```python
from build123d import *

# Parameters (mm, degrees)
BOSS_EXTRUDE1_DEPTH = 13.7
SKETCH3_W           = 0.178571672
SKETCH3_H           = 6.380917094
CUT_EXTRUDE1_DEPTH  = 0.2
SKETCH4_R           = 0.85
BOSS_EXTRUDE3_DEPTH = 1.8
SKETCH5_W           = 0.138137893
SKETCH5_H           = 1.329179466
BOSS_EXTRUDE4_DEPTH = 2.8
SKETCH6_R           = 0.20198457
CUT_EXTRUDE2_DEPTH  = 9.6


with BuildPart() as part:
    # Sketch1 → Boss-Extrude1 (new body)
    with BuildSketch(Plane.XY):
        with BuildLine():
            Line((-3.31662479, -5), (3.31662479, -5))
            ThreePointArc((3.31662479, -5), (6, 0), (3.31662479, 5))
            Line((3.31662479, 5), (-3.31662479, 5))
            ThreePointArc((-3.31662479, 5), (-6, 0), (-3.31662479, -5))
        make_face()
    extrude(amount=BOSS_EXTRUDE1_DEPTH)

    # Sketch3 → Cut-Extrude1 (cut)
    with BuildSketch(Plane(origin=(0, 5, 0), x_dir=(1, 0, 0), z_dir=(0, 1, 0))):
        with Locations((-2.495957535, -5.684471075)):
            Rectangle(SKETCH3_W, SKETCH3_H)
        with Locations((2.495957535, -5.684471075)):
            Rectangle(SKETCH3_W, SKETCH3_H)
    extrude(amount=-CUT_EXTRUDE1_DEPTH, mode=Mode.SUBTRACT)

    # Sketch4 → Boss-Extrude3 (add)
    with BuildSketch(Plane(origin=(0, 0, 0), x_dir=(-1, 0, 0), z_dir=(0, 0, -1))):
        with Locations(Location((0, 0, 0), (0, 0, 180))):
            Circle(SKETCH4_R)
    extrude(amount=BOSS_EXTRUDE3_DEPTH)

    # Sketch5 → Boss-Extrude4 (add)
    with BuildSketch(Plane(origin=(0, 0, 0), x_dir=(-1, 0, 0), z_dir=(0, 0, -1))):
        with Locations((-4.217525365, 0)):
            Rectangle(SKETCH5_W, SKETCH5_H)
        with Locations((4.217525365, 0)):
            Rectangle(SKETCH5_W, SKETCH5_H)
    extrude(amount=BOSS_EXTRUDE4_DEPTH)

    # Sketch6 → Cut-Extrude2 (cut)
    with BuildSketch(Plane.ZY.offset(4.286594311)):
        with Locations((-2.171650698, 0)):
            Circle(SKETCH6_R)
    extrude(amount=-CUT_EXTRUDE2_DEPTH, mode=Mode.SUBTRACT)


solid = part.part
```
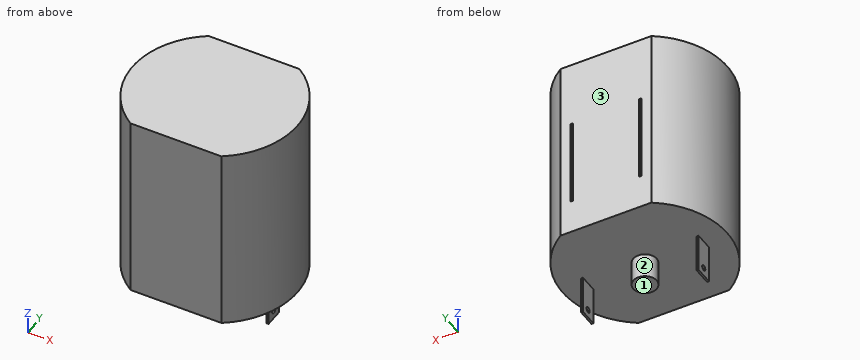
The listing builds one solid part. Answer for the finished solid, in the listing's coordinates (mm). Face numbers are marked on the shaded views. A direction names the side the tool comes from. Coordinates: 2 decimals unless noted, no trailing zeros. Loops run counter-clockwise (first coordinate to the right, second up) from the corner with the lowest first, then second, coordinate; pieces in that order, holes last. Notation, with made-up numbers: (-29, -17) - (-9, -17) arc R28 cw to (-9, 22) - close; hole circle Ø5 at (-35, 17). An arc over 180 degrees is marked (long way). Use a Markdown table: item, result. Add a question column.
1) Find the intervals of material crossed by line 1 (Z direction, x = 0, y = -3); line 2 (Y direction, x = 5, z = 3.5); line 3 (X direction, y = -3.5, z = 6), in increasing order.
2) The part is cut by section A-A, the plane y = 0. Give the vertices of the cut face in (x, z), and give its area (3 significant figures).
3) The part is cut by section B-B, the plane x = 0. Give the vertices of the cut face in (y, z).
4) The part is cut by section C-C, the plane z = 5.25. Give the vertices of the cut face in (x, y), and give its area (3 significant figures).
5) The part is cut by section D-D, the plane y = -1.5. Give the vertices of the cut face in (x, z).
6) For the marked faces 1, 2 and 3, determine the directions among +Z, -Z, +X, -X, +Y, -Y from which every point of the face is accessible in a straight line to the end or side of a thin tool.
7) Given pin 1 (1 mm diameter, centred on x = -3, y = -1.5, fed in from -Z); pin 2 (1.1 mm diameter, centred on y = 0, z = -1, fed in from +X); pin 3 (5 mm diameter, centred on x = -1, y = -0.5, fed in from -Z), each flat-ended and moving along its own axis, determine where each tip first touches the part or whether it passes through.
Here are the results:
| question | item | result |
|---|---|---|
| 1 | line 1 | z = 0 to 13.7 |
| 1 | line 2 | y = -3.32 to 3.32 |
| 1 | line 3 | x = -4.87 to 4.87 |
| 2 | outline | (-6, 0) - (-4.29, 0) - (-4.29, -1.97) - (-4.15, -1.97) - (-4.15, 0) - (-0.85, 0) - (-0.85, -1.8) - (0.85, -1.8) - (0.85, 0) - (4.15, 0) - (4.15, -1.97) - (4.29, -1.97) - (4.29, 0) - (6, 0) - (6, 13.7) - (-6, 13.7) - close; (-4.29, -2.8) - (-4.15, -2.8) - (-4.15, -2.37) - (-4.29, -2.37) - close; (4.15, -2.8) - (4.29, -2.8) - (4.29, -2.37) - (4.15, -2.37) - close |
| 2 | area | 168 mm^2 |
| 3 | outline | (-5, 0) - (-0.85, 0) - (-0.85, -1.8) - (0.85, -1.8) - (0.85, 0) - (5, 0) - (5, 13.7) - (-5, 13.7) - close |
| 4 | outline | (-3.32, -5) - (3.32, -5) arc R6 ccw to (3.32, 5) - (2.59, 5) - (2.59, 4.8) - (2.41, 4.8) - (2.41, 5) - (-2.41, 5) - (-2.41, 4.8) - (-2.59, 4.8) - (-2.59, 5) - (-3.32, 5) arc R6 ccw to start |
| 4 | area | 104 mm^2 |
| 5 | outline | (-5.81, 0) - (5.81, 0) - (5.81, 13.7) - (-5.81, 13.7) - close |
| 6 | face 1 | -Z, +Y, -Y |
| 6 | face 2 | -Z |
| 6 | face 3 | +Z, -Z, +X, -X, +Y |
| 7 | pin 1 | stops at z = 0 |
| 7 | pin 2 | stops at x = 4.29 |
| 7 | pin 3 | stops at z = -1.8 |
